Can you work these out from the drawing? Everything is in mm from the part's minimum corner. Round coordinates to 2 decimals unless told otherwise and drop trailing zeros. Order: outer loops, then holes, each group sorted by start corner. A loop starts at its lowest first (then second) coordinate and runs counter-clockwise, first axis right, second up. Notation, with made-up numbers: (-20.75, -12) -> (6.25, -12) arc R18 ccw to (6.25, 7) -> close; hole circle Ø1 at (-10, 26.25). An arc over 180 degrees is marked (long way). One line per item, written item: value.
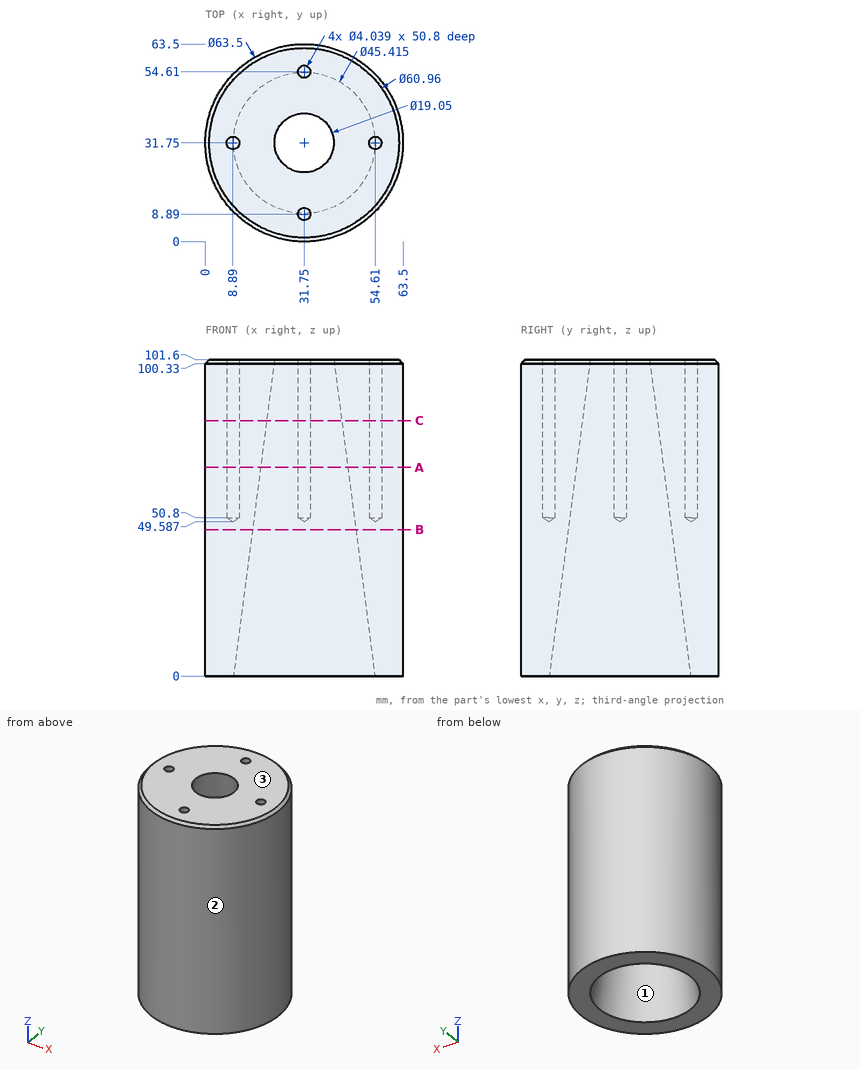
Q1. I want a section at B-B on z = 47. Write out the boundary of the cut face in (x, y).
Answers:
outline: circle Ø63.5 at (31.75, 31.75); hole circle Ø33.22 at (31.75, 31.75)
Q2. If we mould it in two halves opening along Y, with no side actions, what happens to the marked faces 1, 2 and 3? For each: pulls with the +Y half, pulls with the -Y half, needs draft (parallel to the pull), parting line crosses it, or undercut.
Answers:
face 1: undercut
face 2: parting line crosses it
face 3: needs draft
Q3. For P1, Ø1, axis at x = 17, z = 28, coming from the +Y side; P2, Ø1, axis at x = 37, z = 79.5, coming from the -Y side; P3, Ø6, axis at y = 49.5, z = 64.5, coming from the +X side (1 decimal); P4, Ø4.5, axis at x = 54.61, y = 31.75, coming from the +Z side, each with a flat end and sliding along its axis, tell me the tip position at first contact or that it passes through.
Answers:
P1: y = 60.12
P2: y = 0.36
P3: x = 59.9
P4: z = 101.6
Q4. I want a section at C-C on z = 82. Write out the boundary of the cut face in (x, y).
Answers:
outline: circle Ø63.5 at (31.75, 31.75); hole circle Ø4.04 at (8.89, 31.75); hole circle Ø24.14 at (31.75, 31.75); hole circle Ø4.04 at (31.75, 8.89); hole circle Ø4.04 at (31.75, 54.61); hole circle Ø4.04 at (54.61, 31.75)
Q5. I need wall thicknesses on line 1 along X through (y, z) = (31, 67) (1 decimal); line 2 along Y through (x, z) = (32.5, 80.5) (1 decimal); line 3 along X through (y, z) = (32, 81) (1 decimal). Which ranges of each line are inside material? Lowest first, please.
Answers:
line 1: 0 to 7, 10.8 to 17.8, 45.7 to 52.7, 56.5 to 63.5
line 2: 0 to 7, 10.8 to 19.5, 44 to 52.7, 56.5 to 63.5
line 3: 0 to 6.9, 10.9 to 19.6, 43.9 to 52.6, 56.6 to 63.5
Q6. I want a section at A-A on z = 67. Give the number of separate pieces and of enclosed holes in the cut face, then the cut area to 3 significant figures.
Answers:
separate pieces: 1
enclosed holes: 5
area: 2,500 mm2
